Geometry: final body of the model. Coordinates: model frame, mm. Give positions to 0.01 mm unless a question says otherwise; leave off trailing zeros. Loops run counter-clockwise (first coordinate to the right, second up) from the corner with the lowest first, then second, coordinate; pieces in that order, holes last.
1. Section D-D, the plane z = 0.55. Output: boundary loops of the cut face in (x, y).
2. First-contact query: P1, Ø12, axis at x = 12, y = 48.5, coming from the -Z side; P2, Ø0.8, axis at y = 24, z = 1, coming from the +X side. Flat tips, straight axial feed; report the tip coordinate or a pass-through.
3. Material intervals for line 1 along X through (y, z) = (73, 1); line 2 along Y through (x, z) = (2, 1.2); line 3 along X through (y, z) = (53, 0.1), sorted ascending.
4. Section B-B, the plane y = 26. Output: boundary loops of the cut face in (x, z), then the cut area to 3 significant figures.
5. Section A-A, the plane x = -6. Output: boundary loops of the cut face in (y, z), then the cut area to 3 significant figures.
6. Section C-C, the plane y = 73. Output: boundary loops of the cut face in (x, z), then the cut area to 3 significant figures.
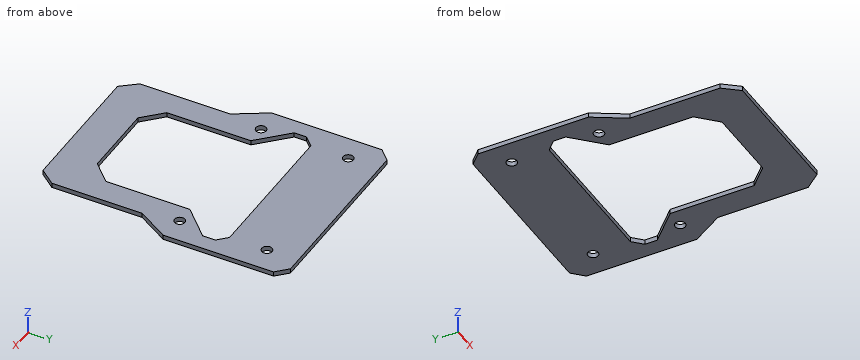
from build123d import *

# Parameters (mm, degrees)
SKETCH_1_R            = 1.65
EXTRUDE_267_DEPTH     = 1.5
SKETCH_3_W            = 200
SKETCH_3_H            = 2
CUT_EXTRUDE_0P5_DEPTH = 1.5


with BuildPart() as part:
    # 草图1 → Extrude 267 (new body)
    with BuildSketch(Plane.XY):
        Polygon((-22, 0), (22, 0), (26, 5), (26, 34), (32, 44), (32, 79.5), (28, 83.5), (-28, 83.5), (-32, 79.5), (-32, 44), (-26, 34), (-26, 5), align=None)
        with Locations((-24, 45)):
            Circle(SKETCH_1_R, mode=Mode.SUBTRACT)
        with Locations((24, 45)):
            Circle(SKETCH_1_R, mode=Mode.SUBTRACT)
        with Locations((-24, 73)):
            Circle(SKETCH_1_R, mode=Mode.SUBTRACT)
        with Locations((24, 73)):
            Circle(SKETCH_1_R, mode=Mode.SUBTRACT)
        Polygon((-24, 61), (24, 61), (27, 58), (27, 54), (18, 45), (18, 18), (12, 12), (-12, 12), (-18, 18), (-18, 45), (-27, 54), (-27, 58), align=None, mode=Mode.SUBTRACT)
    extrude(amount=EXTRUDE_267_DEPTH)

    # 草图3 → 底板加厚上沿退让0p5 (cut)
    with BuildSketch(Plane.XY):
        with Locations((0, 84)):
            Rectangle(SKETCH_3_W, SKETCH_3_H)
    extrude(amount=CUT_EXTRUDE_0P5_DEPTH, mode=Mode.SUBTRACT)


solid = part.part
Answers below:
1. outline: (-32, 44) - (-26, 34) - (-26, 5) - (-22, 0) - (22, 0) - (26, 5) - (26, 34) - (32, 44) - (32, 79.5) - (28.5, 83) - (-28.5, 83) - (-32, 79.5) - close; hole (-27, 54) - (-18, 45) - (-18, 18) - (-12, 12) - (12, 12) - (18, 18) - (18, 45) - (27, 54) - (27, 58) - (24, 61) - (-24, 61) - (-27, 58) - close; hole circle Ø3.3 at (-24, 45); hole circle Ø3.3 at (-24, 73); hole circle Ø3.3 at (24, 45); hole circle Ø3.3 at (24, 73)
2. P1: passes through
2. P2: stops at x = 26
3. line 1: x = -32 to -25.65, -22.35 to 22.35, 25.65 to 32
3. line 2: y = 0 to 12, 61 to 83
3. line 3: x = -32 to -26, 26 to 32
4. outline: (-26, 0) - (-18, 0) - (-18, 1.5) - (-26, 1.5) - close; (18, 0) - (26, 0) - (26, 1.5) - (18, 1.5) - close
4. area: 24.0 mm2
5. outline: (0, 0) - (12, 0) - (12, 1.5) - (0, 1.5) - close; (61, 0) - (83, 0) - (83, 1.5) - (61, 1.5) - close
5. area: 51.0 mm2
6. outline: (-32, 0) - (-25.65, 0) - (-25.65, 1.5) - (-32, 1.5) - close; (-22.35, 0) - (22.35, 0) - (22.35, 1.5) - (-22.35, 1.5) - close; (25.65, 0) - (32, 0) - (32, 1.5) - (25.65, 1.5) - close
6. area: 86.1 mm2
